Design review of the part built by this model. Coordinates are the model's own, in mm. Round coordinates to 2 decimals unless told otherwise and drop trailing zeros. Write each loop counter-clockwise with the first axis right and the second up, starting at its lowest first coordinate (ties: lowest second). Pieces come first, ordered by that corner, then holes. Notation, with made-up numbers: M -32.75,33.5 L -4.75,33.5 A7 cw -4.75,46.5 Z; hole C 86.5,86.5 d7. An arc over 180 degrees is marked long. Use CSV: the item, a comma, the result in double quotes.
from build123d import *

# Parameters (mm, degrees)
F0_R     = 10
F1_DEPTH = 25
F2_DEPTH = 60
F3_SIZE  = 2


with BuildPart() as f1:
    # F0 (on Front) → F1 (new body)
    with BuildSketch(Plane.XZ):
        with BuildLine():
            ThreePointArc((-14.790199, 62.5), (-1.254394, 45.052542), (15, 60))
            ThreePointArc((15, 60), (14.947458, 61.254394), (14.790199, 62.5))
            ThreePointArc((14.790199, 62.5), (0, 75), (-14.790199, 62.5))
        make_face()
        with Locations((0, 60)):
            Circle(F0_R, mode=Mode.SUBTRACT)
        with BuildLine():
            ThreePointArc((14.790199, 62.5), (14.947458, 61.254394), (15, 60))
            ThreePointArc((15, 60), (-1.254394, 45.052542), (-14.790199, 62.5))
            Line((-14.790199, 62.5), (-24.650332, 4.166667))
            ThreePointArc((-24.650332, 4.166667), (0, 25), (24.650332, 4.166667))
            Line((24.650332, 4.166667), (14.790199, 62.5))
        make_face()
        with BuildLine():
            ThreePointArc((25, 0), (24.91243, 2.090657), (24.650332, 4.166667))
            ThreePointArc((24.650332, 4.166667), (0, 25), (-24.650332, 4.166667))
            ThreePointArc((-24.650332, 4.166667), (-2.090657, -24.91243), (25, 0))
        make_face()
        Circle(F0_R, mode=Mode.SUBTRACT)
    extrude(amount=F1_DEPTH)

    # F0 (on Front) → F2 (join)
    with BuildSketch(Plane.XZ):
        with BuildLine():
            ThreePointArc((25, 0), (24.91243, 2.090657), (24.650332, 4.166667))
            ThreePointArc((24.650332, 4.166667), (0, 25), (-24.650332, 4.166667))
            ThreePointArc((-24.650332, 4.166667), (-2.090657, -24.91243), (25, 0))
        make_face()
        Circle(F0_R, mode=Mode.SUBTRACT)
    extrude(amount=F2_DEPTH)

    # F3
    f3_edges = [f1.edges().sort_by_distance(p)[0] for p in [
        (-25, -60, 0),
        (-10, -60, 0),
        (-10, -25, 60),
    ]]
    chamfer(f3_edges, length=F3_SIZE)


solid = f1.part
1) Wall thickness on line 1 along Z through (x, y) = (3.5, -9); line 2 along Z through (x, y) = (-8.5, -7.5); line 3 along Y through (x, z) = (15.5, 54): over which ranges is each line inside the solid? List them lowest first. Write a range as [from, to].
Answers:
line 1,"[-24.75, -9.37], [9.37, 50.63], [69.37, 74.59]"
line 2,"[-23.51, -5.27], [5.27, 54.73], [65.27, 72.36]"
line 3,"[-25, 0]"
2) Add section A-A on x = 0. Write out the cut boundary in (y, z), then the cut area to 3 significant figures.
Answers:
outline,"M -60,-23 L -58,-25 L 0,-25 L 0,-10 L -58,-10 L -60,-12 Z; M -60,12 L -58,10 L 0,10 L 0,50 L -23,50 L -25,48 L -25,25 L -58,25 L -60,23 Z; M -25,72 L -23,70 L 0,70 L 0,75 L -25,75 Z"
area,"2,540 mm²"
3) Add section D-D on y = -40. Write out the cut boundary in (x, z), then the cut area to 3 significant figures.
Answers:
outline,"M 24.65,4.17 A25 ccw long 25,0 A25 ccw Z; hole C 0,0 d20"
area,"1,650 mm²"
4) For pin 1 Ø4 at (y, z) = (-30.5, -9) entering from -X; pin 2 Ø1 at (y, z) = (-17, 49) entering from +X; pin 3 Ø6 at (x, z) = (9.5, 42.5) entering from -Y, all flat-tipped, find the tip position at first contact; note any pin that passes through.
Answers:
pin 1,"x = -24"
pin 2,"x = 17.16"
pin 3,"y = -25"
5) Add section B-B on y = -16. Write out the cut boundary in (x, z), then the cut area to 3 significant figures.
Answers:
outline,"M -24.65,4.17 A25 ccw long 25,0 A25 ccw 24.65,4.17 L 14.79,62.5 A15 ccw -14.79,62.5 Z; hole C 0,0 d20; hole C 0,60 d20"
area,"3,140 mm²"
6) The part is to be moulded in two halves that separate along Z. For faces 1 (the face through (-2.195, -23.125, 50.116)), 2 (the face through (0, -25, 40)), 3 (the face through (-19.65, -12.32, 33.74)), 4 (the face through (-2.17, -11.34, 50.24)), say which applies: released by +Z, released by -Z, zero draft, split by the parting line, or undercut.
Answers:
face 1,"undercut"
face 2,"zero draft"
face 3,"released by +Z"
face 4,"undercut"
7) Add section C-C on z = 60. Write out the cut boundary in (x, y).
Answers:
outline,"M -15.21,-25 L -12,-25 L -10,-23 L -10,0 L -15.21,0 Z; M 10,-23 L 12,-25 L 15.21,-25 L 15.21,0 L 10,0 Z"
